Part print with two shaded views. Sizes in mm from the minimum x, y, z corner. Round coordinates to 2 decimals unless told otherwise and drop trailing zeros. Loops run counter-clockwise (first coordinate to the right, second up) from the corner with the lowest first, then second, coordinate; pieces in that order, holes last.
(1) Cut at A-A on y = 12. List the corners of the cut face in (x, z), then the cut area to 3 significant figures.
(2) Mould opens along Z. For the marked faces 1, 2 and 3 say: +Z half, -Z half, draft (parallel to the pull), parting line (faces both ways), or undercut.
(3) Cut at B-B on z = 102. List the corners of the cut face in (x, y).
(4) Probe probe 1 along X at (y, z) = (7.25, 78). List the from-to ranges inside material, lowest first.
(5) Flat gauge pins, fed straight in: pin 1 (6 mm diameter, centred on x = 342.5, y = 12, fed in from -Z); pin 2 (10 mm diameter, centred on y = 12.5, z = 97, fed in from +X). Where does each tip first touch, or does it go through?
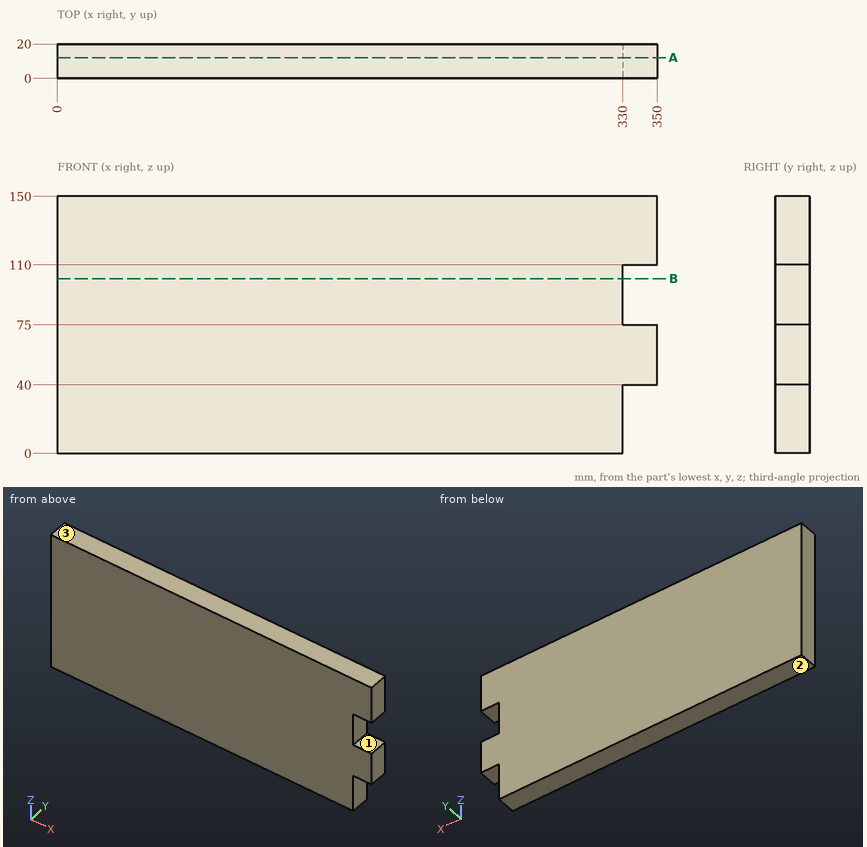
Final values:
1. outline: (0, 0) - (330, 0) - (330, 40) - (350, 40) - (350, 75) - (330, 75) - (330, 110) - (350, 110) - (350, 150) - (0, 150) - close
1. area: 51,000 mm2
2. face 1: undercut
2. face 2: -Z half
2. face 3: +Z half
3. outline: (0, 0) - (330, 0) - (330, 20) - (0, 20) - close
4. probe 1: x = 0 to 330
5. pin 1: stops at z = 40
5. pin 2: stops at x = 330
